The drawing under review shows one solid part. Ordinate dimensions are in mm from its lowest x, y, z. A direction names the side the tool comes from. Coordinates: 2 decimals unless noted, no trailing zeros. Write each loop counter-clockwise with the first axis right and the second up, starting at its lowest first coordinate (ties: lowest second). Pieces come first, ordered by that corner, then holes.
1) We need section C-C on y = 5. Write out the cut boundary in (x, z).
2) We need section D-D on x = 19.37. Write out the cut boundary in (y, z), then the cut area to 3 significant figures.
3) To check wall thickness, follow line 1 along X through (y, z) = (0.8, 11.69) (1 decimal); line 2 along Z through (x, y) = (9.37, 1.15); line 3 along X through (y, z) = (0.65, 16.69). State the ranges of each line that lie inside material, in increasing order.
4) Mouldability with a two-part tool opening along X and no side actions: class the marked faces 3, 4 and 5 as pulls with the +X half, pulls with the -X half, needs draft (parallel to the pull), parting line crosses it, or undercut.
5) We need section B-B on x = 14.37. Write out the cut boundary in (y, z) (1 decimal).
6) Insertion check: P1, Ø1.5, axis at x = 15, z = 13, coming from the +Y side; P2, Ø1.3, axis at x = 1, z = 10.5, coming from the +Y side; P3, Ø11.5, axis at x = 11.5, z = 10, coming from the +Y side. Each pin has a flat end and moves straight along its axis. Give the tip position at first contact, or say it passes through.
7) We need section A-A on z = 11.69. Write out the cut boundary in (x, y) (1 decimal).
8) For the marked faces 1 and 2, list the 3-axis set-ups (+Z, -Z, +X, -X, +Y, -Y) from which the entire face can be reached by the end or side of a thin tool; tool diameter is ignored.
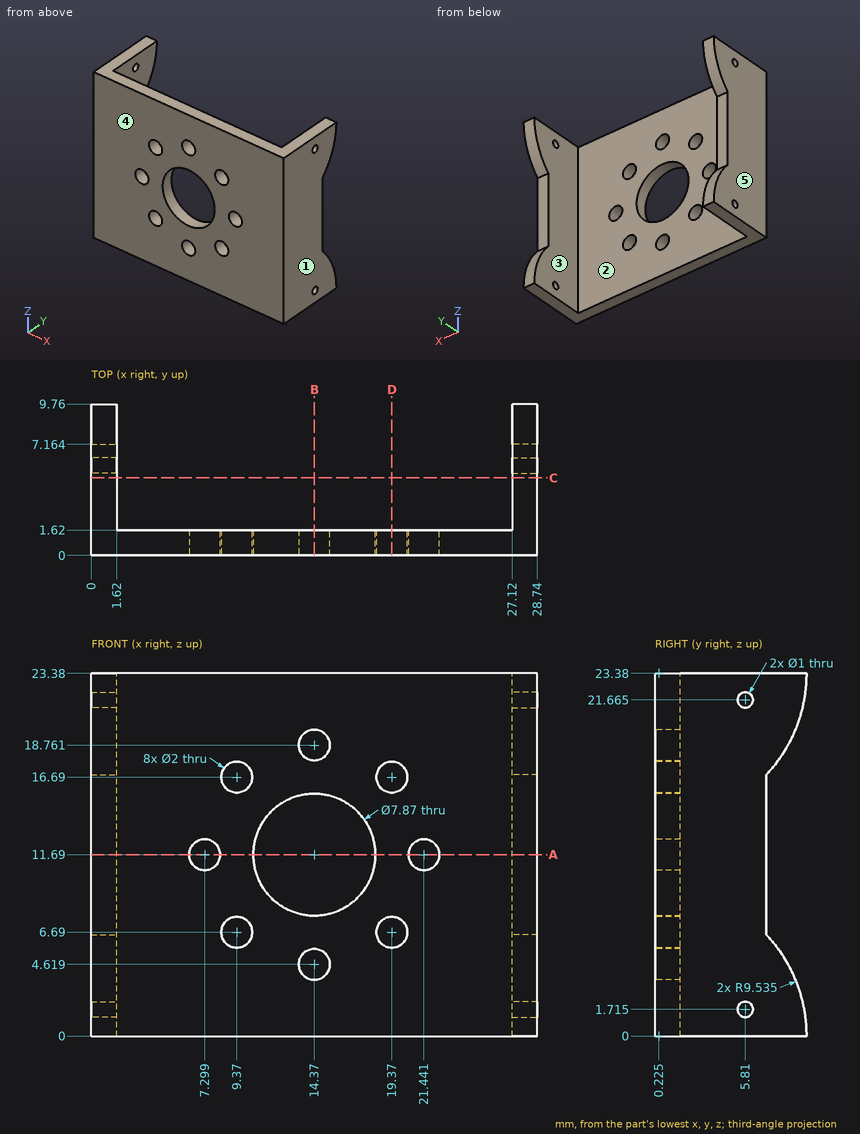
Result:
1. outline: (0, 0) - (1.62, 0) - (1.62, 23.38) - (0, 23.38) - close; (27.12, 0) - (28.74, 0) - (28.74, 23.38) - (27.12, 23.38) - close
2. outline: (0, 0) - (1.62, 0) - (1.62, 5.69) - (0, 5.69) - close; (0, 7.69) - (1.62, 7.69) - (1.62, 15.69) - (0, 15.69) - close; (0, 17.69) - (1.62, 17.69) - (1.62, 23.38) - (0, 23.38) - close
2. area: 31.4 mm2
3. line 1: x = 0 to 6.3, 8.3 to 10.4, 18.3 to 20.4, 22.4 to 28.7
3. line 2: z = 0 to 5.69, 7.69 to 15.69, 17.69 to 23.38
3. line 3: x = 0 to 8.37, 10.37 to 18.37, 20.37 to 28.74
4. face 3: undercut
4. face 4: needs draft
4. face 5: pulls with the -X half
5. outline: (0, 0) - (1.6, 0) - (1.6, 3.6) - (0, 3.6) - close; (0, 5.6) - (1.6, 5.6) - (1.6, 7.8) - (0, 7.8) - close; (0, 15.6) - (1.6, 15.6) - (1.6, 17.8) - (0, 17.8) - close; (0, 19.8) - (1.6, 19.8) - (1.6, 23.4) - (0, 23.4) - close
6. P1: passes through
6. P2: stops at y = 7.16
6. P3: stops at y = 1.62
7. outline: (0, 0) - (6.3, 0) - (6.3, 1.6) - (1.6, 1.6) - (1.6, 7.2) - (0, 7.2) - close; (8.3, 0) - (10.4, 0) - (10.4, 1.6) - (8.3, 1.6) - close; (18.3, 0) - (20.4, 0) - (20.4, 1.6) - (18.3, 1.6) - close; (22.4, 0) - (28.7, 0) - (28.7, 7.2) - (27.1, 7.2) - (27.1, 1.6) - (22.4, 1.6) - close
8. face 1: +Z, -Z, +X, +Y, -Y
8. face 2: +Z, -Z, +Y
